Could you check a few things on this drawing? It's one solid part, dimensions in mm from its lowest x, y, z. A direction names the side the tool comes from. Give positions to 0.01 mm unless a question says otherwise; leave off trailing zeros. Order: outer loops, then holes, each group sorted by start corner. A loop starts at its lowest first (then second) coordinate and runs counter-clockwise, first axis right, second up. Notation, with made-up numbers: (53.5, 64.25) -> (100.5, 64.25) arc R11 ccw to (100.5, 70.25) -> close; hole circle Ø5 at (14, 79). An arc over 180 degrees is marked (long way). Use one line per item in the form item = value. Start each with the question number.
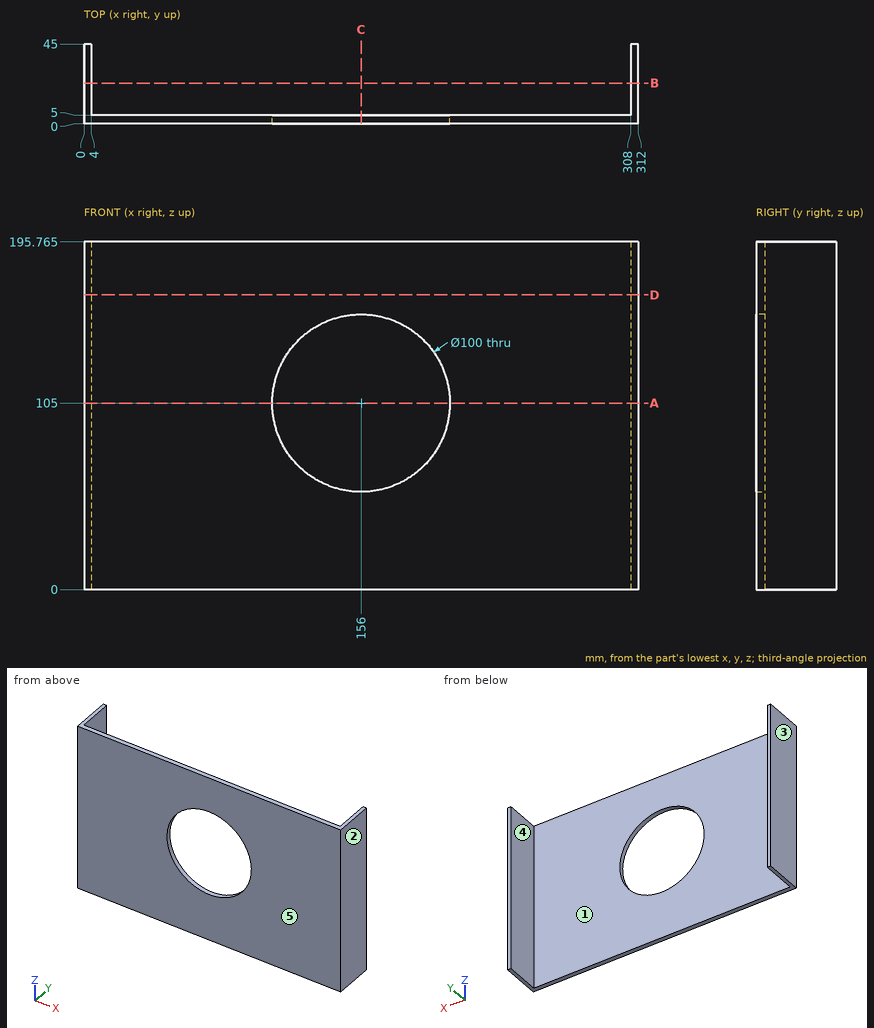
(1) Imagine slicing it at B-B (y = 23). Write out the boundary of the cut face in (x, z) (1 decimal).
(2) Which directions (+Z, -Z, +X, -X, +Y, -Y) give clear straight access to the entire face, cutting with the end or side of a thin tool? Please do the marked faces 4 and 5.
(3) Imagine slicing it at A-A (z = 105). Write out the boundary of the cut face in (x, y), plus the area to 3 significant figures.
(4) Imagine slicing it at C-C (x = 156). Write out the boundary of the cut face in (y, z) (1 decimal).
(5) Please list where these lines run through material, in increasing order: probe 1 along X at (y, z) = (1, 105); probe 2 along X at (y, z) = (8, 90); probe 3 along Y at (x, z) = (38, 114).
(6) I'm going to push a flat-ended pin straight in: pin 1 Ø3 at (x, z) = (45, 140) entering from +Y. Where does the tip first touch, or does it pass through?
(7) Imagine slicing it at D-D (z = 166). Write out the boundary of the cut face in (x, y).
(8) We'd pull the mould along X, two halves only. Please class the marked faces 1, 2 and 3: pulls with the +X half, pulls with the -X half, needs draft (parallel to the pull), parting line crosses it, or undercut.
Calculated:
q1.outline = (0, 0) -> (4, 0) -> (4, 195.8) -> (0, 195.8) -> close; (308, 0) -> (312, 0) -> (312, 195.8) -> (308, 195.8) -> close
q2.face_4 = +Z, -Z, +Y
q2.face_5 = +Z, -Z, +X, -X, -Y
q3.outline = (0, 0) -> (106, 0) -> (106, 5) -> (4, 5) -> (4, 45) -> (0, 45) -> close; (206, 0) -> (312, 0) -> (312, 45) -> (308, 45) -> (308, 5) -> (206, 5) -> close
q3.area = 1,380 mm2
q4.outline = (0, 0) -> (5, 0) -> (5, 55) -> (0, 55) -> close; (0, 155) -> (5, 155) -> (5, 195.8) -> (0, 195.8) -> close
q5.probe_1 = 0 to 106, 206 to 312
q5.probe_2 = 0 to 4, 308 to 312
q5.probe_3 = 0 to 5
q6.pin_1 = 5
q7.outline = (0, 0) -> (312, 0) -> (312, 45) -> (308, 45) -> (308, 5) -> (4, 5) -> (4, 45) -> (0, 45) -> close
q8.face_1 = undercut
q8.face_2 = pulls with the +X half
q8.face_3 = pulls with the -X half
